```python
from build123d import *

# Parameters (mm, degrees)
CROQUIS1_W              = 40
CROQUIS1_H              = 47.3
CROQUIS1_R              = 1
SALIENTE_EXTRUIR1_DEPTH = 30
CROQUIS2_W              = 10
CROQUIS2_H              = 47.3
SALIENTE_EXTRUIR2_DEPTH = 87
CROQUIS3_W              = 17.14601676
CROQUIS3_H              = 47.3
SALIENTE_EXTRUIR3_DEPTH = 30
CROQUIS4_R              = 1
CORTAR_EXTRUIR1_DEPTH   = 118


with BuildPart() as part:
    # Croquis1 → Saliente-Extruir1 (new body)
    with BuildSketch(Plane(origin=(0, 0, 0), x_dir=(0, 0, -1), z_dir=(1, 0, 0))):
        Rectangle(CROQUIS1_W, CROQUIS1_H)
        with Locations((0, 14.489311164)):
            Circle(CROQUIS1_R, mode=Mode.SUBTRACT)
    extrude(amount=SALIENTE_EXTRUIR1_DEPTH)

    # Croquis2 → Saliente-Extruir2 (add)
    with BuildSketch(Plane(origin=(30, 0, 0), x_dir=(0, 0, -1), z_dir=(1, 0, 0))):
        with Locations((-15, 0)):
            Rectangle(CROQUIS2_W, CROQUIS2_H)
    extrude(amount=SALIENTE_EXTRUIR2_DEPTH)

    # Croquis3 → Saliente-Extruir3 (add)
    with BuildSketch(Plane(origin=(0, 0, 10), x_dir=(-1, 0, 0), z_dir=(0, 0, -1))):
        with Locations((-108.42699162, 0)):
            Rectangle(CROQUIS3_W, CROQUIS3_H)
    extrude(amount=SALIENTE_EXTRUIR3_DEPTH)

    # Croquis4 → Cortar-Extruir1 (cut, through all)
    with BuildSketch(Plane.ZY):
        with Locations((0, 14.489311164)):
            Circle(CROQUIS4_R)
    extrude(amount=-CORTAR_EXTRUIR1_DEPTH, mode=Mode.SUBTRACT)


solid = part.part
```
Read the model definition and answer for the solid it produces. Units are mm, in the model's axes. A direction names the side the tool comes from. Coordinates: 2 decimals unless noted, no trailing zeros. Order: outer loops, then holes, each group sorted by start corner. A loop starts at its lowest first (then second) coordinate and runs counter-clockwise, first axis right, second up. Notation, with made-up numbers: (48, -37) - (62, -37) arc R13 cw to (62, -21) - close; hole circle Ø9 at (46.25, -30). An arc over 180 degrees is marked (long way). Answer as a JSON object with one key per item and string values. Group by question number.
Item 1: Consider probe 1 along X at (y, z) = (-18, -17); probe 2 along Y at (x, z) = (9, 0); probe 3 along Z at (x, y) = (84.5, 16.5). Determine where each line is inside the solid, lowest interval first. Write a range as from..to.
Item 2: The mould has two halves that part along Y. Classify faces 3 (the face through (46, 23.65, 14)), 4 (the face through (108.307, 13.513, -0.217)), 5 (the face through (14.79, 13.513, 0.217)), 6 (the face through (46, -23.65, 14)): +Y half, -Y half, draft (parallel to the pull), parting line (faces both ways), or undercut.
Item 3: A tool of negligible diameter and unlimited length cuts with its end or side. For faces 1 (the face through (30, 0, -5)), 2 (the face through (117, 0, 0)), from which of +Z, -Z, +X, -X, +Y, -Y can it reach the whole face along a straight path? Write none if from no direction.
Item 4: Section C-C (x = 62) is taken. Give the vertices of the cut face in (y, z), plus the area to 3 significant figures.
Item 5: Flat-ended cylindrical pins translate along their axes: P1, Ø8, axis at x = 81, y = -14.5, coming from the -Z side; P2, Ø10, axis at x = 39, z = -7.5, coming from the -Y side. Find the tip coordinate at first contact, or state that the pin passes through.
Item 6: Section A-A (z = 4.5) is taken. Give the vertices of the cut face in (x, y), plus the area to 3 significant figures.
Item 7: Section B-B (y = 6) is taken. Give the vertices of the cut face in (x, z), plus the area to 3 significant figures.
Results are:
{
 "1": {"probe 1": "x = 0..30, 99.85..117", "probe 2": "y = -23.65..13.49, 15.49..23.65", "probe 3": "z = 10..20"},
 "2": {"face 3": "+Y half", "face 4": "undercut", "face 5": "undercut", "face 6": "-Y half"},
 "3": {"face 1": "-Z, +Y, -Y", "face 2": "+Z, -Z, +X, +Y, -Y"},
 "4": {"outline": "(-23.65, 10) - (23.65, 10) - (23.65, 20) - (-23.65, 20) - close", "area": "473 mm^2"},
 "5": {"P1": "stops at z = 10", "P2": "passes through"},
 "6": {"outline": "(0, -23.65) - (30, -23.65) - (30, 23.65) - (0, 23.65) - close; (99.85, -23.65) - (117, -23.65) - (117, 23.65) - (99.85, 23.65) - close", "area": "2,230 mm^2"},
 "7": {"outline": "(0, -20) - (30, -20) - (30, 10) - (99.85, 10) - (99.85, -20) - (117, -20) - (117, 20) - (0, 20) - close", "area": "2,580 mm^2"}
}
